Autodesk Inventor part; units mm, degrees
ref_plane "YZ Plane" through (0, 0, 0) normal (1, 0, 0) x (0, 1, 0)
ref_plane "XZ Plane" through (0, 0, 0) normal (0, 1, 0) x (-1, 0, 0)
ref_plane "XY Plane" through (0, 0, 0) normal (0, 0, 1) x (1, 0, 0)
sketch "草图1" plane through (0, 0, 0) normal (0, 1, 0) x (-1, 0, 0)
  line L0 (85, -50) -> (-85, -50)
  line L1 (-90, -45) -> (-90, 45)
  line L2 (-85, 50) -> (85, 50)
  line L3 (90, 45) -> (90, -45)
  line L4 (0, 0) -> (0, -30.3694)
  line L5 (0, 0) -> (-59.6627, 0)
  arc A0 (85, -50) -> (90, -45) centre (85, -45) ccw
  arc A1 (90, 45) -> (85, 50) centre (85, 45) ccw
  arc A2 (-85, 50) -> (-90, 45) centre (-85, 45) ccw
  arc A3 (-90, -45) -> (-85, -50) centre (-85, -45) ccw
  point P0 (90, -50)
  point P1 (-90, 50)
  point P2 (-90, -50)
  dimension "d0" = 180
  dimension "d1" = 100
  dimension "d2" = 5
extrude "拉伸1" add sketch "草图1" along normal blind 4
sketch "草图2" plane through (0, 4, 0) normal (0, 1, 0) x (1, 0, 0)
  line L0 (20, 40.9) -> (10, 40.9)
  line L1 (10, 40.9) -> (10, 30.9)
  line L2 (10, 30.9) -> (20, 30.9)
  line L3 (20, 30.9) -> (20, 40.9)
  line L4 (60, 40.9) -> (70, 40.9)
  line L5 (70, 40.9) -> (70, 30.9)
  line L6 (70, 30.9) -> (60, 30.9)
  line L7 (60, 30.9) -> (60, 40.9)
  line L8 (60, -30.9) -> (70, -30.9)
  line L9 (70, -30.9) -> (70, -40.9)
  line L10 (70, -40.9) -> (60, -40.9)
  line L11 (60, -40.9) -> (60, -30.9)
  line L12 (10, -30.9) -> (20, -30.9)
  line L13 (20, -30.9) -> (20, -40.9)
  line L14 (20, -40.9) -> (10, -40.9)
  line L15 (10, -40.9) -> (10, -30.9)
  line L16 (0, 0) -> (216.0528, 0)
  line L17 (0, 0) -> (0, -71.0339)
  dimension "d5" = 61.8
  dimension "d6" = 10
  dimension "d7" = 10
  dimension "d8" = 40
  dimension "d9" = 20
extrude "拉伸2" add sketch "草图2" along normal blind 30
sketch "草图3" plane through (0, 34, 0) normal (0, 1, 0) x (1, 0, 0)
  line L0 (60, 30.9) -> (70, 30.9)
  line L1 (70, 30.9) -> (70, 40.9)
  line L2 (70, 30.9) -> (70, 40.9)
  line L3 (10, 40.9) -> (10, 30.9)
  line L4 (70, 40.9) -> (10, 40.9)
  line L5 (10, 40.9) -> (10, 30.9)
  line L6 (10, -30.9) -> (10, -40.9)
  line L7 (60, -40.9) -> (70, -40.9)
  line L8 (10, -40.9) -> (70, -40.9)
  line L9 (70, -30.9) -> (70, -40.9)
  line L10 (70, -40.9) -> (70, -30.9)
  line L11 (70, 40.9) -> (70, 30.9)
  line L12 (70, 30.9) -> (70, 22.9)
  line L13 (70, 22.9) -> (10, 22.9)
  line L14 (10, 22.9) -> (10, 30.9)
  line L15 (70, -40.9) -> (70, -30.9)
  line L16 (70, -30.9) -> (70, -22.9)
  line L17 (70, -22.9) -> (10, -22.9)
  line L18 (10, -22.9) -> (10, -30.9)
  point P0 (0, 0)
  dimension "d14" = 18
  dimension "d15" = 18
extrude "拉伸3" add sketch "草图3" along normal blind 5
sketch "草图4" plane through (0, 39, 0) normal (0, 1, 0) x (1, 0, 0)
  line L0 (70, 40.9) -> (10, 40.9)
  line L1 (10, 40.9) -> (70, 40.9)
  line L2 (70, 40.9) -> (70, 31.9)
  line L3 (70, 22.9) -> (70, 40.9)
  line L4 (70, 31.9) -> (10, 31.9)
  line L5 (10, 31.9) -> (10, 40.9)
  line L6 (70, -30.9) -> (70, -40.9)
  line L7 (10, -22.9) -> (10, -40.9)
  line L8 (70, -40.9) -> (10, -40.9)
  line L9 (10, -40.9) -> (10, -31.9)
  line L10 (10, -31.9) -> (70, -31.9)
  line L11 (70, -31.9) -> (70, -40.9)
  point P0 (0, 0)
extrude "拉伸4" add sketch "草图4" along normal blind 9
sketch "草图5" plane through (0, 48, 0) normal (0, 1, 0) x (1, 0, 0)
  line L0 (10, 40.9) -> (20, 40.9)
  line L1 (10, 30.9) -> (10, 22.9)
  line L2 (10, 40.9) -> (10, 22.9)
  line L3 (70, 22.9) -> (70, 30.9)
  line L4 (10, 22.9) -> (70, 22.9)
  line L5 (70, 40.9) -> (70, 30.9)
  line L6 (70, 22.9) -> (70, 40.9)
  line L7 (70, 40.9) -> (10, 40.9)
  line L8 (10, -22.9) -> (70, -22.9)
  line L9 (70, -40.9) -> (60, -40.9)
  line L10 (70, -22.9) -> (70, -40.9)
  line L11 (20, -40.9) -> (10, -40.9)
  line L12 (70, -40.9) -> (10, -40.9)
  line L13 (10, -40.9) -> (10, -22.9)
  point P0 (0, 0)
extrude "拉伸5" add sketch "草图5" along normal blind 4
sketch "草图6" plane through (0, 4, 0) normal (0, 1, 0) x (1, 0, 0)
  line L0 (-73, 28) -> (-73, 16)
  line L1 (-73, 16) -> (-53, 16)
  line L2 (-53, 16) -> (-53, 28)
  line L3 (-53, 28) -> (-73, 28)
  line L4 (-90, 45) -> (-90, -45)
  line L5 (85, 50) -> (-85, 50)
  point P0 (0, 0)
  dimension "d20" = 17
  dimension "d21" = 20
  dimension "d22" = 12
  dimension "d23" = 22
extrude "拉伸6" add sketch "草图6" along normal blind 29
sketch "草图7" plane through (0, 33, 0) normal (0, 1, 0) x (1, 0, 0)
  line L0 (-53, 28) -> (-53, 16)
  line L1 (-53, 28) -> (-53, 16)
  line L2 (-53, 16) -> (-57.5, 16)
  line L3 (-53, 16) -> (-73, 16)
  line L4 (-57.5, 16) -> (-57.5, 28)
  line L5 (-53, 28) -> (-73, 28)
  line L6 (-57.5, 28) -> (-53, 28)
  line L7 (-73, 16) -> (-73, 28)
  line L8 (-73, 28) -> (-73, 16)
  line L9 (-73, 16) -> (-68.5, 16)
  line L10 (-68.5, 16) -> (-68.5, 28)
  line L11 (-73, 28) -> (-68.5, 28)
  point P0 (0, 0)
  dimension "d26" = 4.5
  dimension "d27" = 4.5
extrude "拉伸7" add sketch "草图7" along normal blind 13 contours L0 L2 L4 L5 | L10 L3 L7 L5
sketch "草图8" plane through (0, 4, 0) normal (0, 1, 0) x (1, 0, 0)
  line L0 (-73, -21) -> (-53, -21)
  line L1 (-73, 16) -> (-68.5, 16)
  line L2 (-73, -21) -> (-73, -16)
  line L3 (-73, -16) -> (-53, -16)
  line L4 (-53, -16) -> (-53, -21)
  line L5 (-73, 28) -> (-73, 16)
  point P0 (0, 0)
  dimension "d30" = 37
  dimension "d31" = 5
  dimension "d32" = 20
extrude "拉伸8" add sketch "草图8" along normal blind 45
sketch "草图9" plane through (-73, 4, 21) normal (0, 0, 1) x (1, 0, 0)
  circle A0 centre (10, 35.099) radius 3.6
  line L0 (20, 45) -> (0, 45)
  line L1 (10, 45) -> (10, 16.6489)
  line L2 (-12, 0) -> (158, 0)
  point P0 (73, -4)
  dimension "d35" = 7.2
  dimension "d36" = 35.099
extrude "拉伸9" cut sketch "草图9" against normal blind 10
sketch "草图10" plane through (-73, 4, 16) normal (-1, 0, 0) x (0, 0, 1)
  line L0 (0.0194, -1.086) -> (0.0194, 15)
  line L1 (0.0194, 15) -> (-8.9806, -1.086)
  line L2 (-8.9806, -1.086) -> (0.0194, -1.086)
  line L3 (5.1314, -1.086) -> (14.1314, -1.086)
  line L4 (14.1314, -1.086) -> (5, 15)
  line L5 (5, 15) -> (5, 0)
  line L6 (5, 0) -> (13.5149, 0)
  point P0 (-16, -4)
  dimension "d39" = 9
  dimension "d40" = 9
  dimension "d41" = 15
extrude "拉伸11" add sketch "草图10" against normal blind 20
properties part number "机架"
The model under review builds one solid part; all positions refer to its coordinate system, in mm. A direction names the side the tool comes from. Round coordinates to 2 decimals unless told otherwise and drop trailing zeros. Order: outer loops, then holes, each group sorted by start corner. A loop starts at its lowest first (then second) coordinate and runs counter-clockwise, first axis right, second up.
(1) Wall thickness on L1, parallel to Z at x = 68, y = 38.5; L2, parallel to X at y = 37.5, z = -26; L3, parallel to Y at x = -63, z = 19: over which ranges is each line inside the solid? List them lowest first.
Working result:
L1: z = -40.9 to -22.9, 22.9 to 40.9
L2: x = -73 to -68.5, -57.5 to -53, 10 to 70
L3: y = 0 to 35.5, 42.7 to 49
(2) Take a section at B-B, the plane y = 26.5. State the section outline as (x, z) points.
Working result:
outline: (-73, -28) - (-53, -28) - (-53, -16) - (-73, -16) - close; (-73, 16) - (-53, 16) - (-53, 21) - (-73, 21) - close; (10, -40.9) - (20, -40.9) - (20, -30.9) - (10, -30.9) - close; (10, 30.9) - (20, 30.9) - (20, 40.9) - (10, 40.9) - close; (60, -40.9) - (70, -40.9) - (70, -30.9) - (60, -30.9) - close; (60, 30.9) - (70, 30.9) - (70, 40.9) - (60, 40.9) - close
(3) Take a section at C-C, the plane x = -63. State the section outline as (y, z) points.
Working result:
outline: (0, -50) - (4, -50) - (4, -28) - (33, -28) - (33, -16) - (4, -16) - (4, 7.63) - (18.97, 16) - (35.5, 16) - (35.5, 21) - (19, 21) - (4, 29.51) - (4, 50) - (0, 50) - close; (42.7, 16) - (49, 16) - (49, 21) - (42.7, 21) - close
(4) Mouldability with a two-part tool opening along Z and no side actions: class faces 1 (the face through (1, 2, 50)), 2 (the face through (40, 43, -31.9)), 3 (the face through (-63, 20, -28)) as released by +Z, released by -Z, zero draft, split by the parting line, or undercut.
Working result:
face 1: released by +Z
face 2: undercut
face 3: released by -Z
(5) Tool access review of faces 4 (the face through (20, 19, -36)), 5 (the face through (10, 28, 34)), 6 (the face through (40, 34, 32)), 7 (the face through (40, 43, 31.9)): name each direction out of +Z, -Z, +X, -X, +Y, -Y from which nothing blocks a thin tool from reaching the whole face with its end or side.
Working result:
face 4: +Z, -Z
face 5: +Z, -Z, -X, +Y
face 6: none
face 7: +X, -X
(6) For P1, Ø14.5, axis at x = 40.5, y = 28, coming from the -Z side; P2, Ø3.5, axis at x = -71.5, z = -19.5, coming from the +Y side; P3, Ø5, axis at x = -67, y = 20, coming from the +Z side, all flat-tipped, find the tip position at first contact; note any pin that passes through.
Working result:
P1: stops at z = -40.9
P2: stops at y = 46
P3: stops at z = 21.85
(7) Take a section at A-A, the plane z = 34.5. State the section outline as (x, y) points, plus the area to 3 significant figures.
Working result:
outline: (-90, 0) - (90, 0) - (90, 4) - (70, 4) - (70, 52) - (10, 52) - (10, 4) - (-90, 4) - close; hole (20, 4) - (60, 4) - (60, 34) - (20, 34) - close
area: 2,400 mm2
(8) Take a section at D-D, the plane x = 72.5. State the section outline as (y, z) points, plus the area to 3 significant figures.
Working result:
outline: (0, -50) - (4, -50) - (4, 50) - (0, 50) - close
area: 400 mm2
